Verification items for the finished model (mm, model axes). A direction names the side the tool comes from. Give positions to 0.01 mm unless a question says otherwise; leave off trailing zeros. Loops run counter-clockwise (first coordinate to the right, second up) from the corner with the lowest first, then second, coordinate; pieces in that order, holes last. Notation, with made-up numbers: (51, 73) - (89, 73) arc R29 cw to (89, 105) - close; hole circle Ø2 at (24.25, 39.5). An arc over 180 degrees is marked (long way). One line per item, written item: value. Start each with the question number.
1. Scan lines: L1, parallel to Z at x = 153, y = 60; L2, parallel to X at y = 46, z = 9; L3, parallel to Z at x = 247.5, y = 37.5. Record each from-to range of solid material in increasing order. Write a range as [from, to].
2. Sectioned sample at B-B (y = 45.5). Record the cut outline in (x, z).
3. Sectioned sample at A-A (x = 195). Record the cut outline in (y, z).
4. Mould release check, pull along X, two halves, no side actions. Record for faces 6 (the flat face through (253.053, 53.403, 9.955)), 7 (the flat face through (138.219, 35, 25)), 8 (the flat face through (214.419, 33, 12)), 9 (the flat face through (149.445, 35, 29)): pulls with the +X half, pulls with the -X half, needs draft (parallel to the pull), parting line crosses it, or undercut.
5. Access from +Z, -Z, +X, -X, +Y, -Y to the whole of each face (thin tool, end or side, straight path). Record for faces 1 (the flat face through (167.319, 35, 44)), 2 (the flat face through (253.05, 16.28, 10.24)), 3 (the flat face through (290.619, 35, 23)), 4 (the flat face through (263, 35, 32.155)), 5 (the flat face through (205.374, 35, 28)).
6. Sectioned sample at C-C (x = 271.5). Record the cut outline in (y, z) (3 decimals), plus the area to 3 significant figures.
7. Sectioned sample at D-D (z = 9.5). Record the cut outline in (x, y), plus the area to 3 significant figures.
8. Gauge pin test, flat ends, axial feed: pin 1 (14 mm diameter, centred on y = 29.5, z = 45, fed in from +X); pin 2 (16 mm diameter, centred on y = 23.5, z = 11.5, fed in from +X); pin 3 (2 mm diameter, centred on y = 34.5, z = 17, fed in from +X). Record the tip position at first contact, or that the pin passes through.
from build123d import *

# Parameters (mm, degrees)
F0_W     = 152.4
F0_H     = 76.2
F1_DEPTH = 50.8
F3_DEPTH = 76.2
F5_DEPTH = 76.2
F7_DEPTH = 76.2


with BuildPart() as f1:
    # F0 (on Top) → F1 (new body)
    with BuildSketch(Plane.XY):
        with Locations((214.419328, 35.965416)):
            Rectangle(F0_W, F0_H)
    extrude(amount=F1_DEPTH)

    # F2 (on face) → F3 (cut)
    with BuildSketch(Plane.XZ.offset(2.134584)):
        Polygon((181.445256, 50.8), (167.318881, 50.8), (167.318881, 37.91061), (149.444669, 37.91061), (149.444669, 19.171527), (205.37363, 19.171527), (205.37363, 37.91061), (181.445256, 37.91061), align=None)
    extrude(amount=-F3_DEPTH, mode=Mode.SUBTRACT)

    # F4 (on face) → F5 (cut)
    with BuildSketch(Plane.XZ.offset(2.134584)):
        Polygon((290.619328, 50.8), (218.435228, 50.8), (236.032292, 32.15526), (290.619328, 32.15526), align=None)
    extrude(amount=-F5_DEPTH, mode=Mode.SUBTRACT)

    # F6 (on face) → F7 (cut)
    with BuildSketch(Plane.YZ.offset(290.619328)):
        Polygon((9.271001, 20.193001), (23.494998, 0), (48.895001, 0), (58.039002, 20.193001), align=None)
    extrude(amount=-F7_DEPTH, mode=Mode.SUBTRACT)


solid = f1.part
Results are:
1. L1: z = [0, 19.17], [37.91, 50.8]
1. L2: x = [138.22, 214.42]
1. L3: z = [20.19, 32.16]
2. outline: (138.22, 0) - (214.42, 0) - (214.42, 20.19) - (290.62, 20.19) - (290.62, 32.16) - (236.03, 32.16) - (218.44, 50.8) - (181.45, 50.8) - (181.45, 37.91) - (205.37, 37.91) - (205.37, 19.17) - (149.44, 19.17) - (149.44, 37.91) - (167.32, 37.91) - (167.32, 50.8) - (138.22, 50.8) - close
3. outline: (-2.13, 0) - (74.07, 0) - (74.07, 19.17) - (-2.13, 19.17) - close; (-2.13, 37.91) - (74.07, 37.91) - (74.07, 50.8) - (-2.13, 50.8) - close
4. face 6: needs draft
4. face 7: pulls with the -X half
4. face 8: pulls with the +X half
4. face 9: undercut
5. face 1: +Z, +Y, -Y
5. face 2: +X
5. face 3: +Z, -Z, +X, +Y, -Y
5. face 4: +Z, +X, +Y, -Y
5. face 5: +Y, -Y
6. outline: (-2.135, 0) - (23.495, 0) - (9.271, 20.193) - (58.039, 20.193) - (48.895, 0) - (74.065, 0) - (74.065, 32.155) - (-2.135, 32.155) - close
6. area: 1,700 mm^2
7. outline: (138.22, -2.13) - (290.62, -2.13) - (290.62, 16.8) - (214.42, 16.8) - (214.42, 53.2) - (290.62, 53.2) - (290.62, 74.07) - (138.22, 74.07) - close
7. area: 8,840 mm^2
8. pin 1: stops at x = 230.52
8. pin 2: stops at x = 290.62
8. pin 3: stops at x = 214.42
